Source: CAD feature listing. Evaluate the final solid. Frame: model axes, mm. Round coordinates to 2 decimals unless told otherwise and drop trailing zeros. Write each loop counter-clockwise with the first axis right and the second up, starting at its lowest first coordinate (ties: lowest second). Pieces come first, ordered by that corner, then holes. Notation, with made-up numbers: M 87.25,15 L 143.25,15 A5 cw 143.25,21 Z; hole C 34.25,-6 d11. An arc over 180 degrees is marked long. Answer in a Markdown table with one row per item.
Autodesk Inventor part; units mm, degrees
ref_plane "YZ Plane" through (0, 0, 0) normal (1, 0, 0) x (0, 1, 0)
ref_plane "XZ Plane" through (0, 0, 0) normal (0, 1, 0) x (-1, 0, 0)
ref_plane "XY Plane" through (0, 0, 0) normal (0, 0, 1) x (1, 0, 0)
sketch "Sketch2" plane through (0, 0, 0) normal (1, 0, 0) x (0, 1, 0)
  line L0 (166.1125, -46.875) -> (-166.1125, -46.875)
  line L1 (-166.1125, -46.875) -> (-166.1125, 46.875)
  line L2 (-166.1125, 46.875) -> (166.1125, 46.875)
  line L3 (166.1125, 46.875) -> (166.1125, -46.875)
  line L4 (166.1125, -46.875) -> (-166.1125, 46.875) construction
  line L5 (-166.1125, -46.875) -> (166.1125, 46.875) construction
  line L6 (-166.1125, 41.875) -> (-214.1125, 41.875)
  line L7 (-214.1125, 41.875) -> (-214.1125, -43.7)
  line L8 (-214.1125, -43.7) -> (-166.1125, -43.7)
  line L9 (-166.1125, -43.7) -> (-166.1125, 41.875)
  line L10 (166.1125, -46.875) -> (0, -46.875)
  line L11 (0, -46.875) -> (0, -56.875)
  line L12 (0, -56.875) -> (166.1125, -56.875)
  line L13 (166.1125, -56.875) -> (166.1125, -46.875)
  line L14 (0, 0) -> (0, -46.875)
  line L15 (-166.1125, 46.875) -> (-169.2875, 46.875)
  line L16 (-169.2875, 46.875) -> (-169.2875, 41.875)
  line L17 (-169.2875, 41.875) -> (-166.1125, 41.875)
  line L18 (-166.1125, 41.875) -> (-166.1125, 46.875)
  line L19 (-214.1125, 41.875) -> (-171.6688, 41.875)
  line L20 (-171.6688, 41.875) -> (-171.6688, 46.875)
  line L21 (-171.6688, 46.875) -> (-214.1125, 46.875)
  line L22 (-214.1125, 46.875) -> (-214.1125, 41.875)
  line L23 (-214.1125, 46.875) -> (-173.6687, 46.875)
  line L24 (-173.6687, 46.875) -> (-173.6687, 51.875)
  line L25 (-173.6687, 51.875) -> (-214.1125, 51.875)
  line L26 (-214.1125, 51.875) -> (-214.1125, 46.875)
  line L27 (-171.6688, 46.875) -> (-173.6687, 51.875)
  line L28 (-166.1125, -46.875) -> (0, -46.875)
  line L29 (0, -46.875) -> (0, -48.4625)
  line L30 (0, -48.4625) -> (-166.1125, -48.4625)
  line L31 (-166.1125, -48.4625) -> (-166.1125, -46.875)
  line L32 (0, -56.875) -> (-166.1125, -48.4625)
  dimension "d0" = 332.225
  dimension "d1" = 93.75
  dimension "d6" = 3.175
  dimension "d7" = 5
  dimension "d8" = 48
  dimension "d9" = 10
  dimension "d17" = 0
  dimension "d18" = 3.175
  dimension "d19" = 2.3813
  dimension "d20" = 5
  dimension "d21" = 2
  dimension "d22" = 1.5875
extrude "Extrusion1" add sketch "Sketch2" along normal blind 3.15 contours L13 L12 L11 L0 | L0 L1 L2 L3 | L11 L30 L31 L0 | L11 L32 L30 | L8 L7 L6 L1
sketch "Sketch3" plane through (3.15, 0, 0) normal (1, 0, 0) x (0, 0, -1)
  line L0 (56.875, 0) -> (56.875, 166.1125)
  line L1 (56.875, 166.1125) -> (-46.875, 166.1125)
  line L2 (43.725, 166.1125) -> (46.875, 166.1125)
  line L3 (46.875, 166.1125) -> (46.875, 126.1125)
  line L4 (46.875, 126.1125) -> (43.725, 126.1125)
  line L5 (43.725, 126.1125) -> (43.725, 166.1125)
  line L6 (-41.875, -166.1125) -> (-41.875, -214.1125)
  line L7 (-41.875, -214.1125) -> (43.7, -214.1125)
  circle A0 centre (-26.8187, -190.1125) radius 2.5
  line L8 (48.4625, -166.1125) -> (-41.875, -166.1125)
  line L9 (-41.875, -166.1125) -> (-41.875, -214.1125)
  line L10 (-41.875, -214.1125) -> (48.4625, -214.1125)
  line L11 (48.4625, -214.1125) -> (48.4625, -166.1125)
  line L12 (3.2938, -214.1125) -> (3.2938, -166.1125)
  circle A1 centre (33.4063, -190.1125) radius 2.5
  point P0 (0, 0)
  point P1 (-41.875, -169.2875)
  point P2 (-41.875, -171.6688)
  dimension "d11" = 40
  dimension "d12" = 3.15
  dimension "d13" = 10
  dimension "d23" = 5
  dimension "d24" = 24
  dimension "d25" = 30.1125
extrude "Extrusion2" cut sketch "Sketch3" against normal blind 10 contours L3 L4 L5 L1 | A0 | A1
equation "\"d0\" = window_z"
equation "\"d1\" = window_y"
equation "\"d6\" = 2 * sm_thickness"
equation "\"d7\" = acrylic_into_frame"
equation "\"d8\" = window_overlap"
equation "\"d9\" = protection_slot_width"
equation "\"d18\" = 2 * sm_thickness"
equation "\"d19\" = 1.5 * sm_thickness"
equation "\"d22\" = sm_thickness"
equation "\"d2\" = clear_acrylic"
equation "\"d11\" = 0.5 * protection_slot_length"
equation "\"d12\" = clear_acrylic"
equation "\"d13\" = protection_slot_width"
equation "\"d23\" = m5_diameter"
equation "\"d24\" = 0.5 * window_overlap"
equation "\"d25\" = 0.333333 * drawer_y"
equation "\"sm_thickness\" = 1.5875"
equation "\"very_thick_acrylic\" = 9.45"
equation "\"thick_acrylic\" = 5.88"
equation "\"thin_acrylic\" = 3.15"
equation "\"clear_acrylic\" = 3.15"
equation "\"wood_thickness\" = 6.72"
equation "\"m3_diameter\" = 3"
equation "\"m4_diameter\" = 4"
equation "\"m5_diameter\" = 5"
equation "\"brass_insert_drill\" = 4"
equation "\"m5_brass_insert_drill\" = 6.7"
equation "\"m3_main_length\" = 14"
equation "\"m3_main_nut_width\" = 5.7"
equation "\"m3_main_nut_thickness\" = 2.5"
equation "\"m3_main_extra\" = 1"
equation "\"stepper_screw_space\" = 35"
equation "\"stepper_shaft_diameter\" = 5"
equation "\"stepper_body_diameter\" = 28"
equation "\"laser_body_diameter\" = 12"
equation "\"carrier_y\" = 251"
equation "\"carrier_z\" = 12"
equation "\"visor_x\" = 253.925"
equation "\"visor_y\" = 85.6"
equation "\"protection_slot\" = 44.2"
equation "\"protection_slot_offset\" = 55.25"
equation "\"window_z\" = 332.225"
equation "\"tray_border\" = 25"
equation "\"bed_z\" = 25"
equation "\"reservoir_x\" = 201"
equation "\"crane_z2\" = 12"
equation "\"tray_y\" = 251"
equation "\"door_sensor\" = 35"
equation "\"linear_bearing_spacing\" = 271"
equation "\"motor_spacing\" = 337"
equation "\"tray_x\" = 251"
equation "\"reservoir_y\" = 201"
equation "\"window_y\" = 93.75"
equation "\"end_stop_spacing\" = 19"
equation "\"window_overlap\" = 48"
equation "\"door_z\" = 332.225"
equation "\"door_x\" = 251"
equation "\"door_overlap\" = 48"
equation "\"acrylic_into_frame\" = 5"
equation "\"protection_slot_width\" = 10"
equation "\"laser_z_offset\" = 55"
equation "\"galvo_frame_x\" = 66"
equation "\"galvo_frame_z\" = 85"
equation "\"laser_y_offset\" = 19.4"
equation "\"thumb_nut_diameter\" = 7"
equation "\"drawer_y\" = 90.3375"
equation "\"frame_total_z\" = 661.5875"
equation "\"printer_z\" = 289"
equation "\"subframe_y_offset\" = 27.5"
equation "\"frame_bottom_z\" = 275"
equation "\"lcd_y\" = 25"
equation "\"drawer_x\" = 257.3"
equation "\"drawer_z\" = 278.175"
equation "\"drawer_z_from_bottom\" = 25"
equation "\"t_galvo_frame\" = 6.72"
equation "\"laser_z\" = 75"
equation "\"nema17_x\" = 43"
equation "\"thumb_nut_offset_y\" = 0"
equation "\"laser_y\" = 15"
equation "\"frame_tilt\" = 1deg"
equation "\"frame_top_z\" = 385"
equation "\"frame_border\" = 48.0375"
equation "\"laser_diameter\" = 12"
equation "\"galvo_frame_y_offset\" = 27.5"
equation "\"lcd_x\" = 72"
equation "\"subframe_x\" = 66"
equation "\"frame_foot_z\" = 12"
equation "\"z_min_from_center\" = 115"
equation "\"m3_press_nut_drill\" = 4.5"
equation "\"m3_head\" = 6"
equation "\"m5_head\" = 10.3"
equation "\"m5_press_nut_drill\" = 6.5"
equation "\"drawer_support_from_top\" = 48"
equation "\"laser_gap\" = 1"
equation "\"frame_screw_from_center\" = 25"
equation "\"drawer_screw_from_center\" = 55"
equation "\"frame_face_y\" = 45"
equation "\"switch_spacing\" = 19"
equation "\"subframe_y\" = 55"
equation "\"al_thickness\" = 1.5875"
equation "\"rivet_diameter\" = 3.3"
equation "\"bend_factor\" = 2.26205"
equation "\"sm_bend\" = 3.591"
equation "\"al_bend\" = 3.591"
equation "\"frame_x\" = 353.375"
equation "\"carrier_z2\" = 25"
equation "\"carrier_y2\" = 76.825"
properties part number "window"
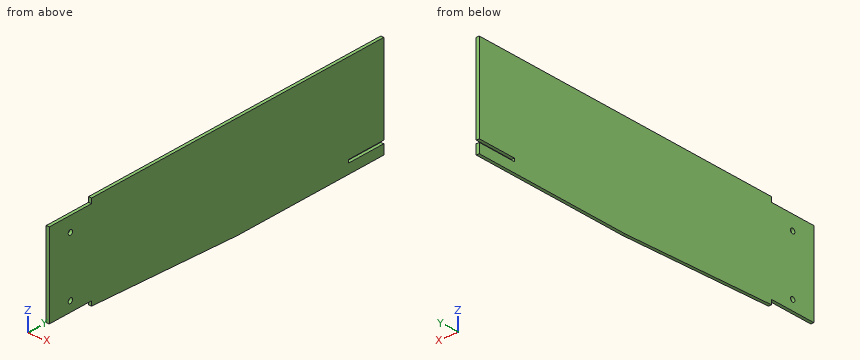
Q1. Material intervals for probe 1 along Y at (x, z) = (0.45, -33); probe 2 along Y at (x, z) = (2.75, 27.5); probe 3 along Z at (x, y) = (0.25, -87) (3 decimals), sorted ascending.
Solutions:
| item | result |
|---|---|
| probe 1 | y = -214.11 to -192.58, -187.65 to 166.11 |
| probe 2 | y = -214.11 to -192.52, -187.71 to 166.11 |
| probe 3 | z = -52.469 to 46.875 |
Q2. Contact query for flat-ended pins moving along their axis: pin 1 Ø6 at (y, z) = (-190.11, 26.82) entering from +X; pin 2 Ø0.9 at (x, z) = (1, 45) entering from -Y; pin 3 Ø0.9 at (x, y) = (1.5, -189.5) entering from +Z (3 decimals); pin 4 Ø1 at (x, y) = (1, -131.5) entering from -Z. Output: stop coordinate, or through.
Solutions:
| item | result |
|---|---|
| pin 1 | stops at x = 3.15 |
| pin 2 | stops at y = -166.11 |
| pin 3 | stops at z = 41.875 |
| pin 4 | stops at z = -50.24 |
Q3. Section A-A (x = 1.8). Return loops of the section in (y, z) (1 decimal), and give its area (3 significant figures).
Solutions:
| item | result |
|---|---|
| outline | M -214.1,-43.7 L -166.1,-43.7 L -166.1,-48.5 L 0,-56.9 L 166.1,-56.9 L 166.1,-46.9 L 126.1,-46.9 L 126.1,-43.7 L 166.1,-43.7 L 166.1,46.9 L -166.1,46.9 L -166.1,41.9 L -214.1,41.9 Z; hole C -190.1,-33.4 d5; hole C -190.1,26.8 d5 |
| area | 37,700 mm2 |
